Read the model definition and answer for the solid it produces. Units are mm, in the model's axes. Face numbers are marked on the shaded views. A direction names the side the tool comes from. Round coordinates to 2 decimals unless told otherwise and drop trailing zeros. Order: outer loops, then holes, each group sorted by start corner. A loop starts at its lowest first (then second) coordinate and runs counter-clockwise, first axis right, second up. Notation, with made-up numbers: (62, -18.75) -> (121, -18.75) arc R31 ccw to (121, 8.25) -> close; hole circle Ø7 at (-9, 32). An arc over 180 degrees is marked (long way). Use a Markdown table: item, result. Add a question column.
1. Consider L1, parallel to Y at x = -12, z = 16.5 (3 decimals); L2, parallel to Z at x = 37, y = 26.5; L3, parallel to X at y = -9.5, z = 28. Determine where each line is inside the solid, lowest interval first. Write a range as [from, to].
2. The mould has two halves that part along Y. Classify the marked faces 1, 2, 3 and 4: +Y half, -Y half, draft (parallel to the pull), parting line (faces both ways), or undercut.
3. Section C-C, the plane x = 12 is taken. Give the vertices of the cut face in (y, z), then the cut area to 3 significant figures.
4. For the marked faces 5, 6, 7 and 8, determine the directions among +Z, -Z, +X, -X, +Y, -Y from which every point of the face is accessible in a straight line to the end or side of a thin tool.
5. Section A-A, the plane y = 26 is taken. Give the vertices of the cut face in (x, z) (3 decimals).
6. Given pin 1 (12.5 mm diameter, centred on x = 61.5, z = 8.5, fed in from -Y); pin 2 (10 mm diameter, centred on x = 39, y = 8.5, fed in from +Z); pin 3 (3 mm diameter, centred on x = -15, y = 35, fed in from +Z), each flat-ended and moving along its own axis, determine where each tip first touches the part or whether it passes through.
7. Section B-B, the plane z = 14 is taken. Give the vertices of the cut face in (x, y) (3 decimals).
8. Section D-D, the plane y = 2 is taken. Give the vertices of the cut face in (x, z), then the cut area to 3 significant figures.
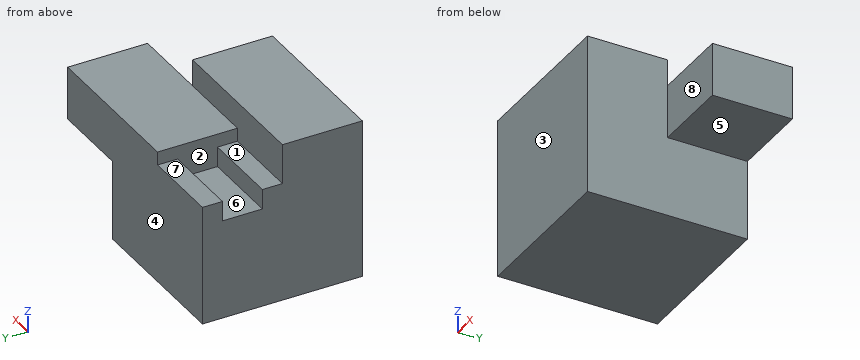
```python
from build123d import *

# Parameters (mm, degrees)
F0_W     = 76.2
F0_H     = 76.2
F1_DEPTH = 38.1
F2_W     = 19.05
F2_H     = 19.05
F3_DEPTH = 38.1
F4_W     = 76.2
F4_H     = 38.1
F5_DEPTH = 19.05
F6_W     = 76.2
F6_H     = 38.1
F7_DEPTH = 25.4


with BuildPart() as f1:
    # F0 (on Top) → F1 (new body, symmetric)
    with BuildSketch(Plane.XY):
        Rectangle(F0_W, F0_H)
    extrude(amount=F1_DEPTH, both=True)

    # F2 (on Right) → F3 (cut)
    with BuildSketch(Plane.YZ):
        with Locations((19.05, 19.05)):
            Rectangle(F2_W, F2_H)
    extrude(amount=-F3_DEPTH, mode=Mode.SUBTRACT)

    # F4 (on face) → F5 (cut)
    with BuildSketch(Plane.XY.offset(38.1)):
        with Locations((0, 19.05)):
            Rectangle(F4_W, F4_H)
    extrude(amount=-F5_DEPTH, mode=Mode.SUBTRACT)

    # F6 (on Top) → F7 (join)
    with BuildSketch(Plane.XY):
        with Locations((38.1, 19.05)):
            Rectangle(F6_W, F6_H)
    extrude(amount=F7_DEPTH)


solid = f1.part
```
Verdict:
| question | item | result |
|---|---|---|
| 1 | L1 | y = [-38.1, 9.525], [28.575, 38.1] |
| 1 | L2 | z = [-38.1, 25.4] |
| 1 | L3 | x = [-38.1, 38.1] |
| 2 | face 1 | draft |
| 2 | face 2 | undercut |
| 2 | face 3 | -Y half |
| 2 | face 4 | +Y half |
| 3 | outline | (-38.1, -38.1) -> (38.1, -38.1) -> (38.1, 25.4) -> (0, 25.4) -> (0, 38.1) -> (-38.1, 38.1) -> close |
| 3 | area | 5,320 mm2 |
| 4 | face 5 | -Z, +X, +Y, -Y |
| 4 | face 6 | +Z, -X |
| 4 | face 7 | +Z, -X, +Y |
| 4 | face 8 | +Z, -Z, +X, -Y |
| 5 | outline | (-38.1, -38.1) -> (38.1, -38.1) -> (38.1, 0) -> (76.2, 0) -> (76.2, 25.4) -> (0, 25.4) -> (0, 9.525) -> (-38.1, 9.525) -> close |
| 6 | pin 1 | stops at y = 0 |
| 6 | pin 2 | stops at z = 25.4 |
| 6 | pin 3 | stops at z = 19.05 |
| 7 | outline | (-38.1, -38.1) -> (38.1, -38.1) -> (38.1, 0) -> (76.2, 0) -> (76.2, 38.1) -> (-38.1, 38.1) -> (-38.1, 28.575) -> (0, 28.575) -> (0, 9.525) -> (-38.1, 9.525) -> close |
| 8 | outline | (-38.1, -38.1) -> (38.1, -38.1) -> (38.1, 0) -> (76.2, 0) -> (76.2, 25.4) -> (0, 25.4) -> (0, 19.05) -> (-38.1, 19.05) -> close |
| 8 | area | 5,560 mm2 |
